from build123d import *

# Parameters (mm, degrees)
F1_DEPTH = 0.8
F2_DEPTH = 35
F3_DEPTH = 15
F4_DEPTH = 5
F5_W     = 30
F5_H     = 1.6
F6_DEPTH = 1.6


with BuildPart() as f1:
    # F0 (on Front) → F1 (new body)
    with BuildSketch(Plane.XZ):
        Polygon((64.041778, -30), (64.041778, 45.94555), (41.6, 29.144735), (41.6, -30), align=None)
        Polygon((1.6, -0.800871), (0, -1.998695), (0, -28.4), (1.6, -28.4), align=None)
        Polygon((1.6, -28.4), (0, -28.4), (0, -30), (40, -30), (40, -28.4), align=None)
        Polygon((64.041778, 47.944246), (0, 0), (0, -1.998695), (1.6, -0.800871), (40, 27.94691), (41.6, 29.144735), (64.041778, 45.94555), align=None)
        Polygon((41.6, -30), (41.6, 29.144735), (40, 27.94691), (40, -28.4), (40, -30), align=None)
        Polygon((40, 27.94691), (1.6, -0.800871), (1.6, -28.4), (40, -28.4), align=None)
    extrude(amount=F1_DEPTH)

    # F0 (on Front) → F2 (join)
    with BuildSketch(Plane.XZ):
        Polygon((1.6, -28.4), (0, -28.4), (0, -30), (40, -30), (40, -28.4), align=None)
    extrude(amount=F2_DEPTH)

    # F0 (on Front) → F3 (join)
    with BuildSketch(Plane.XZ):
        Polygon((64.041778, 47.944246), (0, 0), (0, -1.998695), (1.6, -0.800871), (40, 27.94691), (41.6, 29.144735), (64.041778, 45.94555), align=None)
    extrude(amount=F3_DEPTH)

    # F0 (on Front) → F4 (join)
    with BuildSketch(Plane.XZ):
        Polygon((41.6, -30), (41.6, 29.144735), (40, 27.94691), (40, -28.4), (40, -30), align=None)
        Polygon((1.6, -0.800871), (0, -1.998695), (0, -28.4), (1.6, -28.4), align=None)
    extrude(amount=F4_DEPTH)

    # F5 (on face) → F6 (join)
    with BuildSketch(Plane.YZ.offset(40)):
        with Locations((-20, -29.2)):
            Rectangle(F5_W, F5_H)
        Polygon((-5, 1.6), (-35, -28.4), (-5, -28.4), align=None)
    extrude(amount=F6_DEPTH)


solid = f1.part
Input: part model. Units: mm. Frame: model coordinates. A direction names the side the tool comes from. Round coordinates to 2 decimals unless told otherwise and drop trailing zeros. Write each loop counter-clockwise with the first axis right and the second up, starting at its lowest first coordinate (ties: lowest second). Pieces come first, ordered by that corner, then holes.
1) Cut plane D-D (x = 35.5). Return the cut outline in (y, z), then the cut area to 3 significant figures.
2) Ray query, L1, parallel to X at y = -2, z = -5.5; L2, parallel to Z at x = 9.5, y = -26.5; L3, parallel to Z at x = 10.5, y = -13. Return the intervals inside material, ascending.
3) Draft query along X for faces 5 (the flat face through (39, 0, 1)), 6 (the flat face through (64.042, -0.2, 20.3)), 7 (the flat face through (40, -12, -11)). Return one class per face: pulls with the +X half, pulls with the -X half, needs draft (parallel to the pull), parting line crosses it, or undercut.
4) Cut plane B-B (z = -9.5). Return the cut outline in (x, y).
5) Reachability of faces 1 (the flat face through (0, -4, -16)), 2 (the flat face through (41.6, -10, -13)), 3 (the flat face through (34, -15, 25)), 4 (the flat face through (21, -0.8, -6)) from +Z, -Z, +X, -X, +Y, -Y: full face, straight path, thin tool, end or side. Return the list, or none.
6) Cut plane C-C (y = -32). Return the cut outline in (x, z).
7) Cut plane A-A (y = -11). Return the cut outline in (x, z).
8) Contact query for flat-ended pins moving along their axis: P1, Ø10, axis at x = 40, z = 34.5, coming from the -Y side; P2, Ø6.5, axis at x = 51.5, z = 12.5, coming from the -Y side; P3, Ø0.8, axis at x = 40.5, z = 9.5, coming from the -Y side. Output: stop coordinate, or through.
Geometry says:
1. outline: (-35, -30) - (0, -30) - (0, 26.58) - (-15, 26.58) - (-15, 24.58) - (-0.8, 24.58) - (-0.8, -28.4) - (-35, -28.4) - close
1. area: 128 mm2
2. L1: x = 0 to 1.6, 40 to 41.6
2. L2: z = -30 to -28.4
2. L3: z = -30 to -28.4, 5.86 to 7.86
3. face 5: needs draft
3. face 6: pulls with the +X half
3. face 7: undercut
4. outline: (0, -5) - (1.6, -5) - (1.6, -0.8) - (40, -0.8) - (40, -16.1) - (41.6, -16.1) - (41.6, -0.8) - (64.04, -0.8) - (64.04, 0) - (0, 0) - close
5. face 1: +Z, -Z, -X, +Y, -Y
5. face 2: -Z, +X, -Y
5. face 3: +Z, +X, -X, -Y
5. face 4: -Y
6. outline: (0, -30) - (41.6, -30) - (41.6, -25.4) - (40, -25.4) - (40, -28.4) - (0, -28.4) - close
7. outline: (0, -30) - (41.6, -30) - (41.6, -4.4) - (40, -4.4) - (40, -28.4) - (0, -28.4) - close; (0, -2) - (40, 27.95) - (41.6, 29.14) - (64.04, 45.95) - (64.04, 47.94) - (0, 0) - close
8. P1: stops at y = -15
8. P2: stops at y = -0.8
8. P3: stops at y = -5
